from build123d import *

# Parameters (mm, degrees)
BOX_W           = 10
BOX_H           = 10
BOX_DEPTH       = 10
POCKET_DEPTH    = 0.1
POCKET001_DEPTH = 0.1
POCKET002_DEPTH = 0.1
POCKET003_DEPTH = 0.1
POCKET004_DEPTH = 0.1
SKETCH004_R     = 3.039145
PAD_DEPTH       = 1.2
CHAMFER_SIZE    = 0.5


with BuildPart() as part:
    # Box → Box (new body)
    with BuildSketch(Plane.XY):
        with Locations((5, 5)):
            Rectangle(BOX_W, BOX_H)
    extrude(amount=BOX_DEPTH)

    # Sketch → Pocket (cut)
    with BuildSketch(Plane.XZ):
        with BuildLine():
            ThreePointArc((3.463706, 7.339263), (4.895207, 5.907762), (6.326707, 7.339263))
            Line((6.326707, 7.339263), (6.326707, 9.957689))
            Line((3.463706, 9.957689), (6.326707, 9.957689))
            Line((3.463706, 7.339263), (3.463706, 9.957689))
        make_face()
        with BuildLine():
            ThreePointArc((2.138992, 7.339263), (4.895207, 4.583048), (7.651421, 7.339263))
            Line((7.651421, 7.339263), (7.651421, 9.957689))
            Line((7.651421, 9.957689), (8.879433, 9.957689))
            Line((8.879433, 7.339263), (8.879433, 9.957689))
            ThreePointArc((0.91098, 7.339263), (4.895207, 3.355036), (8.879433, 7.339263))
            Line((0.91098, 7.339263), (0.91098, 9.957689))
            Line((0.91098, 9.957689), (2.138992, 9.957689))
            Line((2.138992, 7.339263), (2.138992, 9.957689))
        make_face()
        with BuildLine():
            ThreePointArc((2.138992, 2.99885), (4.895207, 2.197677), (7.651421, 2.99885))
            Line((7.651421, 2.99885), (7.651421, 1.770838))
            ThreePointArc((2.138992, 1.770838), (4.895207, 1.126045), (7.651421, 1.770838))
            Line((2.138992, 1.770838), (2.138992, 2.99885))
        make_face()
    extrude(amount=-POCKET_DEPTH, mode=Mode.SUBTRACT)

    # Sketch002 → Pocket001 (cut)
    with BuildSketch(Plane(origin=(0, 0, 0), x_dir=(0, -1, 0), z_dir=(-1, 0, 0))):
        with BuildLine():
            ThreePointArc((-4.81849, 0), (-6.828268, 2.9025), (-9.934856, 4.579648))
            Line((-9.934856, 6.139799), (-9.934856, 4.579648))
            ThreePointArc((-3.211477, 0), (-5.749594, 3.971752), (-9.934856, 6.139799))
            Line((-4.81849, 0), (-3.211477, 0))
        make_face()
        with BuildLine():
            ThreePointArc((-1.643138, 0), (-4.681073, 5.034844), (-9.934856, 7.676145))
            Line((-9.934856, 9.258963), (-9.934856, 7.676145))
            ThreePointArc((-0.036126, 0), (-3.575905, 6.136466), (-9.934856, 9.258963))
            Line((-1.643138, 0), (-0.036126, 0))
        make_face()
        with BuildLine():
            ThreePointArc((-0.036126, 3.448501), (-2.553846, 6.82983), (-5.999368, 9.258963))
            Line((-5.999368, 9.258963), (-3.910095, 9.258963))
            ThreePointArc((-0.036126, 5.459331), (-1.792647, 7.543141), (-3.910095, 9.258963))
            Line((-0.036126, 3.448501), (-0.036126, 5.459331))
        make_face()
    extrude(amount=-POCKET001_DEPTH, mode=Mode.SUBTRACT)

    # MirroredSketch → Pocket002 (cut)
    with BuildSketch(Plane.YZ.offset(10)):
        with BuildLine():
            ThreePointArc((9.934856, 4.579648), (6.828268, 2.9025), (4.81849, 0))
            Line((4.81849, 0), (3.211477, 0))
            ThreePointArc((9.934856, 6.139799), (5.749594, 3.971752), (3.211477, 0))
            Line((9.934856, 6.139799), (9.934856, 4.579648))
        make_face()
        with BuildLine():
            ThreePointArc((9.934856, 7.676145), (4.681073, 5.034844), (1.643138, 0))
            Line((1.643138, 0), (0.036126, 0))
            ThreePointArc((9.934856, 9.258963), (3.575905, 6.136466), (0.036126, 0))
            Line((9.934856, 9.258963), (9.934856, 7.676145))
        make_face()
        with BuildLine():
            ThreePointArc((5.999368, 9.258963), (2.553846, 6.82983), (0.036126, 3.448501))
            Line((0.036126, 3.448501), (0.036126, 5.459331))
            ThreePointArc((3.910095, 9.258963), (1.792647, 7.543141), (0.036126, 5.459331))
            Line((5.999368, 9.258963), (3.910095, 9.258963))
        make_face()
    extrude(amount=-POCKET002_DEPTH, mode=Mode.SUBTRACT)

    # Sketch003 → Pocket003 (cut)
    with BuildSketch(Plane(origin=(0, 10, 0), x_dir=(-1, 0, 0), z_dir=(0, 1, 0))):
        with BuildLine():
            Line((-9.999658, -0.012374), (-8.643554, -0.012374))
            Line((-8.643554, -0.012374), (-8.643554, 1.995852))
            ThreePointArc((-8.643554, 1.995852), (-8.940726, 4.204003), (-9.999658, 6.164336))
            Line((-9.999658, 6.164336), (-9.999658, -0.012374))
        make_face()
        with BuildLine():
            Line((-1.547691, 0), (0, 0))
            Line((0, 0), (0, 6.164336))
            ThreePointArc((0, 6.164336), (-1.204366, 4.239939), (-1.547691, 1.995852))
            Line((-1.547691, 1.995852), (-1.547691, 0))
        make_face()
        with BuildLine():
            Line((-4.104364, 0), (-2.665364, 0))
            Line((-2.665364, 0), (-2.665364, 1.995852))
            ThreePointArc((0, 7.654373), (-2.030261, 5.153697), (-2.665364, 1.995852))
            Line((0, 7.654373), (0, 9.37382))
            ThreePointArc((0, 9.37382), (-3.079716, 6.256453), (-4.104364, 1.995852))
            Line((-4.104364, 1.995852), (-4.104364, 0))
        make_face()
        with BuildLine():
            Line((-7.616147, 0), (-6.260043, 0))
            Line((-6.260043, 0), (-6.260043, 1.995852))
            ThreePointArc((-6.260043, 1.995852), (-7.181906, 6.165314), (-9.999658, 9.37382))
            Line((-9.999658, 9.37382), (-9.999658, 7.654373))
            ThreePointArc((-7.616147, 1.995852), (-8.176765, 5.090964), (-9.999658, 7.654373))
            Line((-7.616147, 1.995852), (-7.616147, 0))
        make_face()
        with BuildLine():
            Line((-6.65638, 9.37382), (-5.363037, 9.37382))
            ThreePointArc((-4.944312, 8.776727), (-5.149072, 9.078501), (-5.363037, 9.37382))
            ThreePointArc((-4.482091, 9.37382), (-4.718282, 9.079206), (-4.944312, 8.776727))
            Line((-4.482091, 9.37382), (-3.020288, 9.37382))
            ThreePointArc((-3.020288, 9.37382), (-4.094424, 8.106605), (-4.944312, 6.679266))
            ThreePointArc((-4.944312, 6.679266), (-5.700431, 8.090028), (-6.65638, 9.37382))
        make_face()
    extrude(amount=-POCKET003_DEPTH, mode=Mode.SUBTRACT)

    # Sketch001 → Pocket004 (cut)
    with BuildSketch(Plane.XY.offset(10)):
        with BuildLine():
            ThreePointArc((7.634555, 5.18548), (4.891092, 7.928942), (2.14763, 5.18548))
            Line((2.14763, 5.18548), (2.14763, -0.110033))
            Line((0.880684, -0.110033), (2.14763, -0.110033))
            Line((0.880684, 5.18548), (0.880684, -0.110033))
            ThreePointArc((8.901501, 5.18548), (4.891092, 9.195889), (0.880684, 5.18548))
            Line((8.901501, 5.18548), (8.901501, -0.110033))
            Line((7.634555, -0.110033), (8.901501, -0.110033))
            Line((7.634555, 5.18548), (7.634555, -0.110033))
        make_face()
        with BuildLine():
            ThreePointArc((6.297082, 5.18548), (4.891092, 6.591469), (3.485103, 5.18548))
            Line((3.485103, 5.18548), (3.485103, -0.110033))
            Line((3.485103, -0.110033), (6.297082, -0.110033))
            Line((6.297082, 5.18548), (6.297082, -0.110033))
        make_face()
    extrude(amount=-POCKET004_DEPTH, mode=Mode.SUBTRACT)

    # Sketch004 → Pad (new body)
    with BuildSketch(Plane(origin=(0, 0, 0), x_dir=(1, 0, 0), z_dir=(0, 0, -1))):
        with Locations((4.98763, -5.035975)):
            Circle(SKETCH004_R)
    extrude(amount=PAD_DEPTH)

    # Chamfer
    chamfer_edges = [part.edges().sort_by_distance(p)[0] for p in [
        (1.948485, 5.035975, -1.2),
    ]]
    chamfer(chamfer_edges, length=CHAMFER_SIZE)


solid = part.part
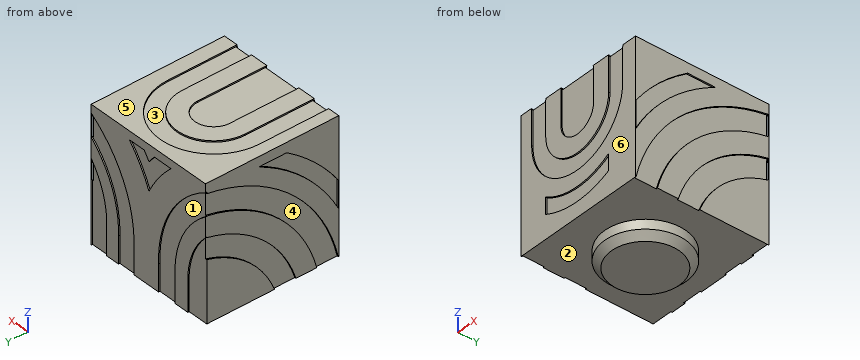
The model under review builds one solid part; all positions refer to its coordinate system, in mm. Face numbers are marked on the shaded views. A direction names the side the tool comes from. Coordinates: 2 decimals unless noted, no trailing zeros. Loops run counter-clockwise (first coordinate to the right, second up) from the corner with the lowest first, then second, coordinate; pieces in that order, holes last. Notation, with made-up numbers: (6, 38) -> (63, 38) arc R22 cw to (63, 69) -> close; hole circle Ø11 at (8, -11.5). An arc over 180 degrees is marked (long way). Use a Markdown table: item, result. Add a question column.
1. To check wall thickness, follow line 1 (Z direction, x = 2, y = 3.5); line 2 (Z direction, x = 4.25, y = 5.25); line 3 (Y direction, x = 4.5, z = 9). State the ranges of each line that lie inside material, in increasing order.
2. Add section B-B on x = 9.25. Write out the cut boundary in (y, z), plus the area to 3 significant figures.
3. Draft analysis for pull direction Z (two halves, no side actions). For the marked faces 4, 5 and 6, state which applies: pulls with the +Z half, pulls with the -Z half, needs draft (parallel to the pull), parting line crosses it, or undercut.
4. Add section A-A on y = 9. Write out the cut boundary in (x, z).
5. Clearance check with a flat-ended pin moving along its axis: pin 1 Ø1.5 at (x, z) = (6.5, 1) entering from -Y. State where the tip first meets the part, or that it passes through.
6. Machinability: for the marked faces 1, 2 and 3, which of the approach directions +Z, -Z, +X, -X, +Y, -Y give a long, thin tool a straight path to every point of the face, cutting with its end or side? Answer none if there is none.
Returned:
| question | item | result |
|---|---|---|
| 1 | line 1 | z = 0 to 9.9 |
| 1 | line 2 | z = -1.2 to 9.9 |
| 1 | line 3 | y = 0.1 to 9.9 |
| 2 | outline | (0, 0) -> (9.9, 0) -> (9.9, 4.97) -> (10, 4.97) -> (10, 6.87) -> (9.9, 6.87) -> (9.9, 8.8) -> (10, 8.8) -> (10, 10) -> (0, 10) -> close |
| 2 | area | 99.3 mm² |
| 3 | face 4 | undercut |
| 3 | face 5 | pulls with the +Z half |
| 3 | face 6 | needs draft |
| 4 | outline | (0, 0) -> (10, 0) -> (10, 4.26) -> (9.9, 4.26) -> (9.9, 5.88) -> (10, 5.88) -> (10, 7.46) -> (9.9, 7.46) -> (9.9, 9.07) -> (10, 9.07) -> (10, 10) -> (6.13, 10) -> (6.13, 9.9) -> (3.65, 9.9) -> (3.65, 10) -> (0, 10) -> (0, 9.07) -> (0.1, 9.07) -> (0.1, 7.46) -> (0, 7.46) -> (0, 5.88) -> (0.1, 5.88) -> (0.1, 4.26) -> (0, 4.26) -> close |
| 5 | pin 1 | stops at y = 0 |
| 6 | face 1 | +Y |
| 6 | face 2 | -Z |
| 6 | face 3 | +Z |
